Geometry: final body of the model. Coordinates: model frame, mm. Give positions to 0.01 mm unless a question says otherwise; leave off trailing zeros. Write each loop counter-clockwise with the first axis right and the second up, starting at its lowest first coordinate (ties: lowest second). Pieces come first, ordered by that corner, then holes. Notation, with made-up numbers: (7.5, 11) -> (41.5, 11) arc R24 cw to (41.5, 50) -> close; hole circle Ø6 at (82, 34.5). An arc over 180 degrees is marked (long way). Answer as a JSON object with one key per item and string values.
from build123d import *

# Parameters (mm, degrees)
F0_R     = 1.55
F0_R_2   = 1.5
F0_R_3   = 20
F1_DEPTH = 4
F2_SIZE  = 1.7


with BuildPart() as f1:
    # F0 (on Right) → F1 (new body)
    with BuildSketch(Plane.YZ):
        with BuildLine():
            ThreePointArc((31.75, 34.25), (31.164214, 35.664214), (29.75, 36.25))
            Line((29.75, 36.25), (-29.75, 36.25))
            ThreePointArc((-29.75, 36.25), (-31.164214, 35.664214), (-31.75, 34.25))
            Line((-31.75, 34.25), (-31.75, -36.25))
            Line((-31.75, -36.25), (31.75, -36.25))
            Line((31.75, -36.25), (31.75, 34.25))
        make_face()
        with Locations((-24.821896, -30.8)):
            Circle(F0_R, mode=Mode.SUBTRACT)
        with Locations((0, -30.75)):
            Circle(F0_R_2, mode=Mode.SUBTRACT)
        with Locations((23.940323, -30.8)):
            Circle(F0_R, mode=Mode.SUBTRACT)
        with Locations((-21.5, 24.58)):
            Circle(F0_R_2, mode=Mode.SUBTRACT)
        with Locations((0, 2.25)):
            Circle(F0_R_3, mode=Mode.SUBTRACT)
        with Locations((0, 30.75)):
            Circle(F0_R, mode=Mode.SUBTRACT)
        with Locations((21.5, 24.58)):
            Circle(F0_R_2, mode=Mode.SUBTRACT)
    extrude(amount=F1_DEPTH)

    # F2
    f2_edges = [f1.edges().sort_by_distance(p)[0] for p in [
        (4, -26.371896, -30.8),
        (4, 22.390323, -30.8),
        (4, -1.55, 30.75),
    ]]
    chamfer(f2_edges, length=F2_SIZE)


solid = f1.part
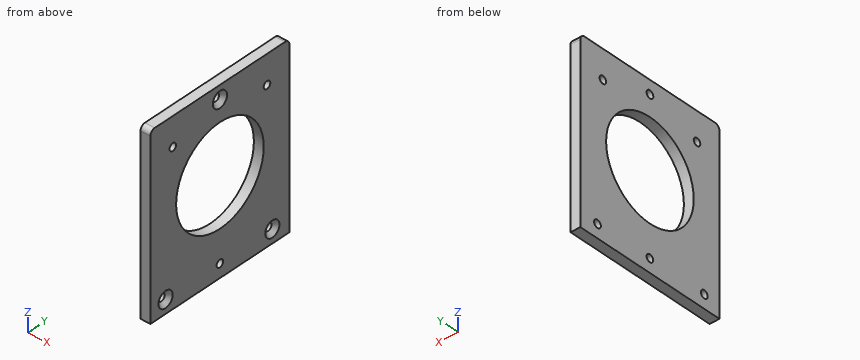
Q1. Cut plane B-B (y = -12.5). Return the cut outline in (x, z), and give its area (3 significant figures).
Values:
{"outline": "(0, -36.25) -> (4, -36.25) -> (4, -13.36) -> (0, -13.36) -> close; (0, 17.86) -> (4, 17.86) -> (4, 36.25) -> (0, 36.25) -> close", "area": "165 mm²"}
Q2. Material intervals for L1, parallel to Z at x = 0.85, y = 0; L2, parallel to Y at x = 2.55, z = 25; L3, parallel to Y at x = 2.6, z = 30.5, sorted ascending. Write a range as from..to.
Values:
{"L1": "-36.25..-32.25, -29.25..-17.75, 22.25..29.2, 32.3..36.25", "L2": "-31.75..-22.94, -20.06..20.06, 22.94..31.75", "L3": "-31.75..-1.83, 1.83..31.75"}
Q3. First-contact query: P1, Ø4, axis at y = -24.82, z = -30.8, coming from the +X side. Flat tip, straight axial feed; report the tip coordinate or a pass-through.
Values:
{"P1": "x = 2.75"}
Q4. Cut plane C-C (x = 0.65). Return the cut outline in (y, z).
Values:
{"outline": "(-31.75, -36.25) -> (31.75, -36.25) -> (31.75, 34.25) arc R2 ccw to (29.75, 36.25) -> (-29.75, 36.25) arc R2 ccw to (-31.75, 34.25) -> close; hole circle Ø3.1 at (-24.82, -30.8); hole circle Ø3 at (-21.5, 24.58); hole circle Ø40 at (0, 2.25); hole circle Ø3.1 at (0, 30.75); hole circle Ø3 at (0, -30.75); hole circle Ø3 at (21.5, 24.58); hole circle Ø3.1 at (23.94, -30.8)"}
Q5. Cut plane A-A (z = 30.75). Return the cut outline in (x, y), and give its area (3 significant figures).
Values:
{"outline": "(0, -31.75) -> (4, -31.75) -> (4, -3.25) -> (2.3, -1.55) -> (0, -1.55) -> close; (0, 1.55) -> (2.3, 1.55) -> (4, 3.25) -> (4, 31.75) -> (0, 31.75) -> close", "area": "239 mm²"}
Q6. Cut plane D-D (z = 2.25). Return the cut outline in (x, y).
Values:
{"outline": "(0, -31.75) -> (4, -31.75) -> (4, -20) -> (0, -20) -> close; (0, 20) -> (4, 20) -> (4, 31.75) -> (0, 31.75) -> close"}
